Could you check a few things on this model? Use its own coordinates, in mm. A direction names the side the tool comes from. Round coordinates to 2 decimals unless told otherwise and drop trailing zeros. Order: outer loops, then holes, each group sorted by start corner. A loop starts at its lowest first (then second) coordinate and runs counter-clockwise, first axis right, second up.
```python
from build123d import *

# Parameters (mm, degrees)
SKETCH1_W           = 30
SKETCH1_H           = 30
SKETCH1_R           = 8.5
BOSS_EXTRUDE1_DEPTH = 6
SKETCH3_R           = 1.5
CUT_EXTRUDE2_DEPTH  = 7
SKETCH4_R           = 3
CUT_EXTRUDE3_DEPTH  = 3
FILLET1_R           = 3


with BuildPart() as part:
    # Sketch1 → Boss-Extrude1 (new body)
    with BuildSketch(Plane.XY):
        Rectangle(SKETCH1_W, SKETCH1_H)
        Circle(SKETCH1_R, mode=Mode.SUBTRACT)
    extrude(amount=BOSS_EXTRUDE1_DEPTH)

    # Sketch3 → Cut-Extrude2 (cut, through all)
    with BuildSketch(Plane.XY.offset(6)):
        with Locations((-11, 11)):
            Circle(SKETCH3_R)
        with Locations((11, 11)):
            Circle(SKETCH3_R)
        with Locations((11, -11)):
            Circle(SKETCH3_R)
        with Locations((-11, -11)):
            Circle(SKETCH3_R)
    extrude(amount=-CUT_EXTRUDE2_DEPTH, mode=Mode.SUBTRACT)

    # Sketch4 → Cut-Extrude3 (cut)
    with BuildSketch(Plane.XY.offset(6)):
        with Locations((-11, 11)):
            Circle(SKETCH4_R)
        with Locations((11, 11)):
            Circle(SKETCH4_R)
        with Locations((11, -11)):
            Circle(SKETCH4_R)
        with Locations((-11, -11)):
            Circle(SKETCH4_R)
    extrude(amount=-CUT_EXTRUDE3_DEPTH, mode=Mode.SUBTRACT)

    # Fillet1
    fillet1_edges = [part.edges().sort_by_distance(p)[0] for p in [
        (15, -15, 3),
        (-15, -15, 3),
        (-15, 15, 3),
        (15, 15, 3),
    ]]
    fillet(fillet1_edges, radius=FILLET1_R)


solid = part.part
```
Q1. Imagine slicing it at A-A, the plane x = 0. Please give me the cut outline in (y, z).
Q2. I need wall thicknesses on L1, parallel to Y at x = -11, z = 5.1; L2, parallel to Y at x = -11, z = 1.35; L3, parallel to Y at x = 0, z = 3.5. Which ranges of each line are inside material? Lowest first, please.
Q3. For faces 1 (the flat face through (12.3, -12.3, 3)), 2 (the cylindrical face through (14.1, -14.14, 3.04)), which set-ups out of +Z, -Z, +X, -X, +Y, -Y let a thin tool reach every point of the face, with its end or its side?
Q4. Imagine slicing it at B-B, the plane y = -11. Please give me the cut outline in (x, z).
Q5. For P1, Ø1.8, axis at x = 10, y = -12, coming from the +Z side; P2, Ø2.5, axis at x = -11, y = -11, coming from the +Z side (1 decimal), each with a flat end and sliding along its axis, tell me the tip position at first contact or that it passes through.
Q6. We'd pull the mould along X, two halves only. Please class faces 3 (the cylindrical face through (-14.14, -14.1, 3.04)), 4 (the flat face through (0, 15, 3)), 5 (the flat face through (15, 0, 3)), 6 (the flat face through (12.3, 9.7, 3)): released by +X, released by -X, zero draft, split by the parting line, or undercut.
Q7. Imagine slicing it at C-C, the plane z = 1.85. Please give me the cut outline in (x, y).
Filled in:
1. outline: (-15, 0) - (-8.5, 0) - (-8.5, 6) - (-15, 6) - close; (8.5, 0) - (15, 0) - (15, 6) - (8.5, 6) - close
2. L1: y = -15 to -14, -8 to 8, 14 to 15
2. L2: y = -15 to -12.5, -9.5 to 9.5, 12.5 to 15
2. L3: y = -15 to -8.5, 8.5 to 15
3. face 1: +Z
3. face 2: +Z, -Z, +X, -Y
4. outline: (-15, 0) - (-12.5, 0) - (-12.5, 3) - (-14, 3) - (-14, 6) - (-15, 6) - close; (-9.5, 0) - (9.5, 0) - (9.5, 3) - (8, 3) - (8, 6) - (-8, 6) - (-8, 3) - (-9.5, 3) - close; (12.5, 0) - (15, 0) - (15, 6) - (14, 6) - (14, 3) - (12.5, 3) - close
5. P1: stops at z = 3
5. P2: passes through
6. face 3: released by -X
6. face 4: zero draft
6. face 5: released by +X
6. face 6: undercut
7. outline: (-15, -12) arc R3 ccw to (-12, -15) - (12, -15) arc R3 ccw to (15, -12) - (15, 12) arc R3 ccw to (12, 15) - (-12, 15) arc R3 ccw to (-15, 12) - close; hole circle Ø3 at (-11, -11); hole circle Ø3 at (-11, 11); hole circle Ø17 at (0, 0); hole circle Ø3 at (11, -11); hole circle Ø3 at (11, 11)
